```python
from build123d import *

# Parameters (mm, degrees)
F0_R     = 7.5
F1_DEPTH = 10
F2_DEPTH = 50
F3_DEPTH = 45


with BuildPart() as f1:
    # F0 (on Front) → F1 (new body)
    with BuildSketch(Plane.XZ):
        Polygon((-25.520833, 11.727427), (-38.020833, -9.923208), (-13.020833, -9.923208), (0, -9.923208), (11.979167, -9.923208), (36.979167, -9.923208), (24.479167, 11.727427), (11.979167, 11.727427), align=None)
        with Locations((-13.020833, 0.90211)):
            Circle(F0_R, mode=Mode.SUBTRACT)
        with Locations((11.979167, 0.90211)):
            Circle(F0_R, mode=Mode.SUBTRACT)
        with BuildLine():
            Line((-119.589004, -9.923208), (-38.020833, -9.923208))
            Line((-38.020833, -9.923208), (-25.520833, 11.727427))
            Line((-25.520833, 11.727427), (-119.425573, 11.727427))
            ThreePointArc((-119.425573, 11.727427), (-119.996581, 0.905803), (-119.589004, -9.923208))
        make_face()
        with BuildLine():
            Line((-149.671407, -9.923208), (-119.589004, -9.923208))
            ThreePointArc((-119.589004, -9.923208), (-119.996581, 0.905803), (-119.425573, 11.727427))
            Line((-119.425573, 11.727427), (-149.540855, 11.727427))
            ThreePointArc((-149.540855, 11.727427), (-149.997273, 0.904468), (-149.671407, -9.923208))
        make_face()
        with Locations((-134.55675, 0.896197)):
            Circle(F0_R, mode=Mode.SUBTRACT)
        with Locations((-134.55675, 0.896197)):
            Circle(F0_R)
    extrude(amount=F1_DEPTH)

    # F0 (on Front) → F2 (join)
    with BuildSketch(Plane.XZ):
        with Locations((-13.020833, 0.90211)):
            Circle(F0_R)
        with Locations((11.979167, 0.90211)):
            Circle(F0_R)
    extrude(amount=F2_DEPTH)

    # F0 (on Front) → F3 (join)
    with BuildSketch(Plane.XZ):
        with Locations((-134.55675, 0.896197)):
            Circle(F0_R)
    extrude(amount=-F3_DEPTH)


solid = f1.part
```
Can you work these out from the model? Positions are in its coordinate system, mm. A direction names the side the tool comes from. Give positions to 0.01 mm unless a question says otherwise; leave off trailing zeros. Order: outer loops, then holes, each group sorted by start corner. A loop starts at its lowest first (then second) coordinate and runs counter-clockwise, first axis right, second up. Notation, with made-up numbers: M -16,19.25 L -4,19.25 A26 ccw -4,38.25 Z; hole C 13,28 d5. An arc over 180 degrees is marked long. One line per item, written item: value.
1) Please list where these lines run through material, in increasing order: line 1 along X through (y, z) = (-23.5, 1); line 2 along Y through (x, z) = (-55, 7); line 3 along Y through (x, z) = (8.5, -5).
Answer sheet:
line 1: x = -20.52 to -5.52, 4.48 to 19.48
line 2: y = -10 to 0
line 3: y = -50 to 0
2) On a 3-axis mill with a long thin cutter (end or side, diameter ignored), from which of +Z, -Z, +X, -X, +Y, -Y can I reach the whole of each face in a straight line? I mean faces 1 (the face through (-18.973, -29.72, -3.662)), 2 (the face through (-142.05, 22.18, 1.23)), 3 (the face through (-149.996, -4.93, 1.056)). Say none if no direction works.
Answer sheet:
face 1: -Y
face 2: +Y
face 3: -X, +Y, -Y
3) I want a section at A-A, the plane z = -2.75. List the corners of the cut face in (x, y) for me.
Answer sheet:
outline: M -149.97,-10 L -19.57,-10 L -19.57,-50 L -6.47,-50 L -6.47,-10 L 5.43,-10 L 5.43,-50 L 18.53,-50 L 18.53,-10 L 32.84,-10 L 32.84,0 L -128,0 L -128,45 L -141.11,45 L -141.11,0 L -149.97,0 Z
4) I want a section at C-C, the plane x = -15. List the corners of the cut face in (y, z) for me.
Answer sheet:
outline: M -50,-6.33 L -10,-6.33 L -10,-9.92 L 0,-9.92 L 0,11.73 L -10,11.73 L -10,8.14 L -50,8.14 Z
5) For P1, Ø12, axis at x = -115.5, z = 6.5, coming from the +Y side; P2, Ø10, axis at y = 13, z = -3.5, coming from the -X side; P3, Ø4, axis at x = 6, y = -29.5, coming from the +Z side, each with a flat end and sliding along its axis, tell me the tip position at first contact or that it passes through.
Answer sheet:
P1: stops at y = 0
P2: stops at x = -142.06
P3: stops at z = 7.26
6) I want a section at D-D, the plane y = -37. List the corners of the cut face in (x, z) for me.
Answer sheet:
outline: C -13.02,0.9 d15; C 11.98,0.9 d15
7) I want a section at B-B, the plane y = -6. List the corners of the cut face in (x, z) for me.
Answer sheet:
outline: M -149.67,-9.92 L 36.98,-9.92 L 24.48,11.73 L -149.54,11.73 A150 ccw Z
